Read the model definition and answer for the solid it produces. Units are mm, in the model's axes. Face numbers are marked on the shaded views. A direction names the side the tool comes from. Coordinates: 2 decimals unless noted, no trailing zeros. Loops run counter-clockwise (first coordinate to the right, second up) from the corner with the lowest first, then second, coordinate; pieces in that order, holes last. Notation, with made-up numbers: (20.5, 63) - (34.5, 63) arc R22 cw to (34.5, 86) - close; hole circle Ø7 at (22, 19). An arc over 180 degrees is marked (long way). Use one line per item in the form item = value.
from build123d import *

# Parameters (mm, degrees)
BOSS_EXTRUDE1_DEPTH     = 20
CUT_EXTRUDE1_DEPTH      = 102.980390272
CUT_EXTRUDE1_DEPTH_BACK = 102.980390272
SKETCH2_R               = 5


with BuildPart() as part:
    # Sketch1 → Boss-Extrude1 (new body)
    with BuildSketch(Plane.XY):
        Polygon((0, 0), (0, 70), (-50, 70), (-50, 0), (-60, 0), (-60, 80), (10, 80), (10, 0), align=None)
    extrude(amount=BOSS_EXTRUDE1_DEPTH)

    # Sketch2 → Cut-Extrude1 (cut, two sides: drawn at the far end of the back side and taken through both)
    with BuildSketch(Plane.ZY.offset(-CUT_EXTRUDE1_DEPTH_BACK)):
        with Locations(Location((10, 15, 0), (0, 0, 180))):
            Circle(SKETCH2_R)
    extrude(amount=CUT_EXTRUDE1_DEPTH + CUT_EXTRUDE1_DEPTH_BACK, mode=Mode.SUBTRACT)


solid = part.part
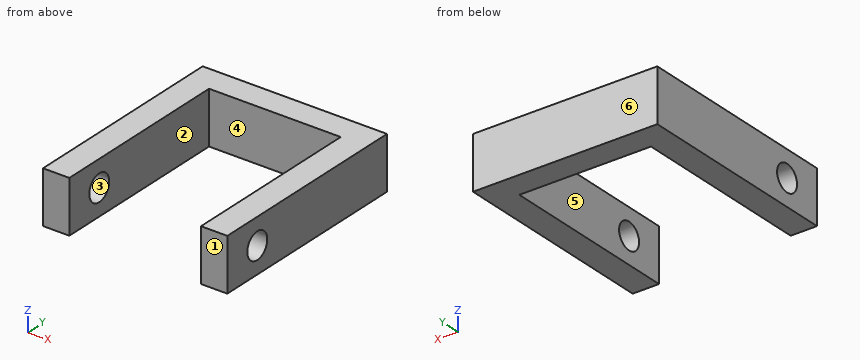
Item 1: The part is cut by section C-C on y = 15. Give the vertices of the cut face in (x, z).
Results below:
outline = (-60, 0) - (-50, 0) - (-50, 5) - (-60, 5) - close; (-60, 15) - (-50, 15) - (-50, 20) - (-60, 20) - close; (0, 0) - (10, 0) - (10, 5) - (0, 5) - close; (0, 15) - (10, 15) - (10, 20) - (0, 20) - close
Item 2: Find the intervals of material crossed by L1, parallel to Y at x = 2.5, z = 10; L2, parallel to X at y = 62.5, z = 2.25; L3, parallel to Y at x = -36, z = 1, in increasing order.
Results below:
L1 = 0 to 10, 20 to 80
L2 = -60 to -50, 0 to 10
L3 = 70 to 80
Item 3: The part is cut by section D-D on z = 18. Give the vertices of the cut face in (x, y), plus the area to 3 significant figures.
Results below:
outline = (-60, 0) - (-50, 0) - (-50, 70) - (0, 70) - (0, 0) - (10, 0) - (10, 80) - (-60, 80) - close
area = 2,100 mm²
Item 4: Which of the six approach directions +Z, -Z, +X, -X, +Y, -Y give full straight-line access (tool end or side, diameter ignored) to the marked faces 1 and 2?
Results below:
face_1 = +Z, -Z, +X, -X, -Y
face_2 = +Z, -Z, -Y
Item 5: For a pull along Y with two mould halves and no side action, classify the marked faces 3, 4, 5 and 6 as +Y half, -Y half, draft (parallel to the pull), parting line (faces both ways), or undercut.
Results below:
face_3 = undercut
face_4 = -Y half
face_5 = draft
face_6 = +Y half
Item 6: The part is cut by section A-A on y = 36. Give the vertices of the cut face in (x, z).
Results below:
outline = (-60, 0) - (-50, 0) - (-50, 20) - (-60, 20) - close; (0, 0) - (10, 0) - (10, 20) - (0, 20) - close
Item 7: This flat-tipped pin is pushed along its axis until it touches: P1, Ø6, axis at x = -18, z = 12, coming from the -Y side. Where does it stop, or does it pass through?
Results below:
P1 = 70
Item 8: The part is cut by section B-B on z = 10. Give the vertices of the cut face in (x, y).
Results below:
outline = (-60, 0) - (-50, 0) - (-50, 10) - (-60, 10) - close; (-60, 20) - (-50, 20) - (-50, 70) - (0, 70) - (0, 20) - (10, 20) - (10, 80) - (-60, 80) - close; (0, 0) - (10, 0) - (10, 10) - (0, 10) - close
